```python
from build123d import *

# Parameters (mm, degrees)
SKETCH1_W           = 158.8
SKETCH1_H           = 53
SKETCH1_R           = 1.4
SKETCH1_R_2         = 1.25
SKETCH1_R_3         = 1.45
BOSS_EXTRUDE1_DEPTH = 220
FILLET1_R           = 5
FILLET2_R           = 5
FILLET3_R           = 5
FILLET4_R           = 5


with BuildPart() as part:
    # Sketch1 → Boss-Extrude1 (new body)
    with BuildSketch(Plane(origin=(0, 0, 0), x_dir=(1, 0, 0), z_dir=(0, 1, 0))):
        with Locations((-25.778590477, -11.5)):
            Rectangle(SKETCH1_W, SKETCH1_H)
        with Locations(Location((-100.664295238, 11, 0), (0, 0, 270))):
            Circle(SKETCH1_R, mode=Mode.SUBTRACT)
        with Locations(Location((48.885704762, 11, 0), (0, 0, 270))):
            Circle(SKETCH1_R_2, mode=Mode.SUBTRACT)
        with Locations(Location((-100.664295238, -33.5, 0), (0, 0, 270))):
            Circle(SKETCH1_R_3, mode=Mode.SUBTRACT)
        with Locations(Location((48.885704762, -33.5, 0), (0, 0, 270))):
            Circle(SKETCH1_R_2, mode=Mode.SUBTRACT)
        Polygon((49, -31), (49, -32), (47.621409523, -32), (47.621409523, -35), (-99.178590477, -35), (-99.178590477, -32), (-99.186141089, -32), (-99.186141089, -31), (-101.006752445, -31), (-101.006752445, -29.2), (-100.997355004, -29.2), (-100.997355004, -4), (-102.15, -4), (-102.15, -2.2), (-101, -2.2), (-101, 2.2), (-102.15, 2.2), (-102.15, 4), (-101, 4), (-101, 6.2), (-102.15, 6.2), (-102.15, 8), (-101, 8), (-101, 9), (-99.178590477, 9), (-99.178590477, 13), (47.621409523, 13), (47.621409523, 9), (49, 9), (49, 8), (50.15, 8), (50.15, -16.8), (49, -16.8), (49, -19), (50.15, -19), (50.15, -20.8), (49, -20.8), (49, -25.2), (50.15, -25.2), (50.15, -27), (49, -27), (49, -29.2), (50.15, -29.2), (50.15, -31), align=None, mode=Mode.SUBTRACT)
    extrude(amount=BOSS_EXTRUDE1_DEPTH)

    # Fillet1
    fillet1_edges = [part.edges().sort_by_distance(p)[0] for p in [
        (-105.178590477, 110, -15),
    ]]
    fillet(fillet1_edges, radius=FILLET1_R)

    # Fillet2
    fillet2_edges = [part.edges().sort_by_distance(p)[0] for p in [
        (-105.178590477, 110, 38),
    ]]
    fillet(fillet2_edges, radius=FILLET2_R)

    # Fillet3
    fillet3_edges = [part.edges().sort_by_distance(p)[0] for p in [
        (53.621409523, 110, -15),
    ]]
    fillet(fillet3_edges, radius=FILLET3_R)

    # Fillet4
    fillet4_edges = [part.edges().sort_by_distance(p)[0] for p in [
        (53.621409523, 110, 38),
    ]]
    fillet(fillet4_edges, radius=FILLET4_R)


solid = part.part
```
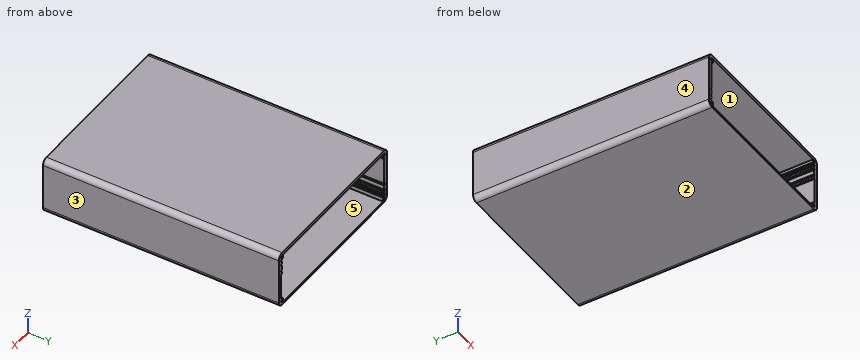
Part model, mm, in its own coordinate system. Face numbers are marked on the shaded views. A direction names the side the tool comes from. Coordinates: 2 decimals unless noted, no trailing zeros. Loops run counter-clockwise (first coordinate to the right, second up) from the corner with the lowest first, then second, coordinate; pieces in that order, holes last. Notation, with made-up numbers: (88, 29.5) - (100, 29.5) arc R17 cw to (100, 52.5) - close; hole circle Ø7 at (51, 79). An arc over 180 degrees is marked (long way). Write item = value, one per line. Start each with the question number.
Item 1: Cut at B-B, the plane x = 24. Give the cut face in (y, z), and give its area (3 significant figures).
Item 2: Flat gauge pins, fed straight in: pin 1 Ø1.3 at (x, y) = (-101.5, 61.5) entering from -Z; pin 2 Ø1.3 at (x, y) = (49.5, 92.5) entering from +Z. Where does each tip first touch, or does it go through?
Item 3: Cut at A-A, the plane z = 13. Give the cut face in (x, y).
Item 4: Cut at C-C, the plane y = 127. State how many separate pieces and enclosed holes the cut face has, and give its area (3 significant figures).
Item 5: Wall check: L1, parallel to X at y = 144, z = 28.5; L2, parallel to X at y = 29, z = -7; L3, parallel to Z at x = -35.5, y = 161. Give the ranges that are in metal, low to high. Write a range as from..to.
Item 6: 3-axis set-ups, long thin cutter, end or side, ignore diameter. For the marked faces 4 and 5: which of +Z, -Z, +X, -X, +Y, -Y reach the whole face in a straight line?
Item 7: Mould opens along X. For the marked faces 1, 2 and 3 say: released by +X, released by -X, zero draft, split by the parting line, or undercut.
The answers:
q1.outline = (0, -15) - (220, -15) - (220, -13) - (0, -13) - close; (0, 35) - (220, 35) - (220, 38) - (0, 38) - close
q1.area = 1,100 mm2
q2.pin_1 = -14.95
q2.pin_2 = 37.99
q3.outline = (-105.18, 0) - (-101, 0) - (-101, 220) - (-105.18, 220) - close; (50.15, 0) - (53.62, 0) - (53.62, 220) - (50.15, 220) - close
q4.separate_pieces = 1
q4.enclosed_holes = 5
q4.area = 1,160 mm2
q5.L1 = -105.18..-101, 49..53.62
q5.L2 = -105.18..-102.15, 50.15..53.62
q5.L3 = -15..-13, 35..38
q6.face_4 = +Z, -Z, -X, +Y, -Y
q6.face_5 = +Y, -Y
q7.face_1 = undercut
q7.face_2 = zero draft
q7.face_3 = released by +X
